Verification items for the finished model (mm, model axes). Face numbers are marked on the shaded views. A direction names the side the tool comes from. Coordinates: 2 decimals unless noted, no trailing zeros. Loops run counter-clockwise (first coordinate to the right, second up) from the corner with the lowest first, then second, coordinate; pieces in that order, holes last. Notation, with made-up numbers: (76.25, 78) -> (124.25, 78) arc R21 cw to (124.25, 106) -> close; hole circle Ø3 at (24, 87.5). An arc over 180 degrees is marked (long way). Write item = value, one per line.
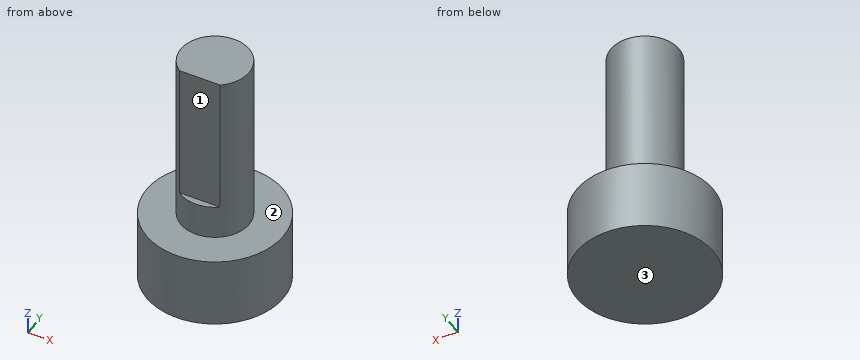
```python
from build123d import *

# Parameters (mm, degrees)
CROQUIS2_R                 = 6
SALIENTE_EXTRUIR1_DEPTH    = 6.2
CROQUIS3_R                 = 3
SALIENTE_EXTRUIR2_DEPTH    = 15.2
CORTAR_EXTRUIR1_DEPTH      = 24.020860106
CORTAR_EXTRUIR1_DEPTH_BACK = 12.2


with BuildPart() as part:
    # Croquis2 → Saliente-Extruir1 (new body)
    with BuildSketch(Plane.XY):
        Circle(CROQUIS2_R)
    extrude(amount=-SALIENTE_EXTRUIR1_DEPTH)

    # Croquis3 → Saliente-Extruir2 (add)
    with BuildSketch(Plane.XY):
        with Locations(Location((0, 0, 0), (0, 0, 180))):
            Circle(CROQUIS3_R)
    extrude(amount=SALIENTE_EXTRUIR2_DEPTH)

    # Croquis4 → Cortar-Extruir1 (cut, two sides: drawn at the far end of the back side and taken through both)
    with BuildSketch(Plane.XY.offset(15.2).offset(-CORTAR_EXTRUIR1_DEPTH_BACK)):
        Polygon((34.725967809, -2.4), (1.8, -2.4), (-1.8, -2.4), (-34.725967809, -2.4), (-34.725967809, -68.251935619), (34.725967809, -68.251935619), align=None)
    extrude(amount=CORTAR_EXTRUIR1_DEPTH + CORTAR_EXTRUIR1_DEPTH_BACK, mode=Mode.SUBTRACT)


solid = part.part
```
1) Sectioned sample at B-B, the plane x = 0. Record the cut outline in (y, z), plus the area to 3 significant figures.
Ans:
outline = (-6, -6.2) -> (6, -6.2) -> (6, 0) -> (3, 0) -> (3, 15.2) -> (-2.4, 15.2) -> (-2.4, 3) -> (-3, 3) -> (-3, 0) -> (-6, 0) -> close
area = 158 mm2
2) Depth check by flat-ended pin: pin 1 Ø5 at (x, z) = (-3.5, 5.5) entering from +Y; pin 2 Ø1.8 at (x, z) = (0.5, 10.5) entering from -Y; pin 3 Ø4 at (y, z) = (-0.5, -1) entering from -X; pin 4 Ø1.5 at (y, z) = (1, 9) entering from +X. Enter the tip coordinate at first touch or a pass-through.
Ans:
pin_1 = 2.83
pin_2 = -2.4
pin_3 = -6
pin_4 = 2.99
3) Material ranges on line 1 (Z direction, x = -0.25, y = -3.5); line 2 (X direction, y = 0.25, z = -3.25); line 3 (X direction, y = -1, z = 0.25), recorded low to high.
Ans:
line_1 = -6.2 to 0
line_2 = -5.99 to 5.99
line_3 = -2.83 to 2.83
4) Sectioned sample at D-D, the plane y = 5.25. Record the cut outline in (x, z).
Ans:
outline = (-2.9, -6.2) -> (2.9, -6.2) -> (2.9, 0) -> (-2.9, 0) -> close
5) Tool access check on the marked faces 1, 2 and 3. Record the directions out of +Z, -Z, +X, -X, +Y, -Y that give a thin tool (end or side, any length) a straight path to the whole face; none if there is none.
Ans:
face_1 = +Z, +X, -X, -Y
face_2 = +Z
face_3 = -Z, +X, -X, +Y, -Y
6) Sectioned sample at A-A, the plane y = 0. Record the cut outline in (x, z).
Ans:
outline = (-6, -6.2) -> (6, -6.2) -> (6, 0) -> (3, 0) -> (3, 15.2) -> (-3, 15.2) -> (-3, 0) -> (-6, 0) -> close
7) Sectioned sample at C-C, the plane z = 1.5. Record the cut outline in (x, y).
Ans:
outline = circle Ø6 at (0, 0)
